The listing builds one solid part. Answer for the finished solid, in the listing's coordinates (mm). Face numbers are marked on the shaded views. Round coordinates to 2 decimals unless told otherwise and drop trailing zeros. Write each loop counter-clockwise with the first axis right and the second up, starting at its lowest first coordinate (ties: lowest second). Pieces come first, ordered by that corner, then holes.
Item 1: Find section A-A on z = 0. Give the vertices of the cut face in (x, y).
Item 2: Find section B-B on x = 0. Give the vertices of the cut face in (y, z).
Item 3: Find section C-C on y = -23. Give the vertices of the cut face in (x, z), then the cut area to 3 significant figures.
Item 4: Find section D-D on x = 38. Give the vertices of the cut face in (y, z), then the cut area to 3 significant figures.
Item 5: For a pull along Z with two mould halves and no side action, classify the marked faces 1, 2 and 3 as +Z half, -Z half, draft (parallel to the pull), parting line (faces both ways), or undercut.
Item 6: Find the intervals of material crossed by probe 1 along Z at (x, y) = (0, -11.5); probe 2 along Z at (x, y) = (-5.5, -10.5); probe 3 along X at (y, z) = (-4.5, 9), in increasing order.
Item 7: Each of these flat-tipped pins is pushed along its axis until it touches: pin 1 (4 mm diameter, centred on y = -19, z = 28, fed in from -X); pin 2 (3 mm diameter, centred on y = -14.5, z = 28, fed in from +X). Where does it stop, or does it pass through?
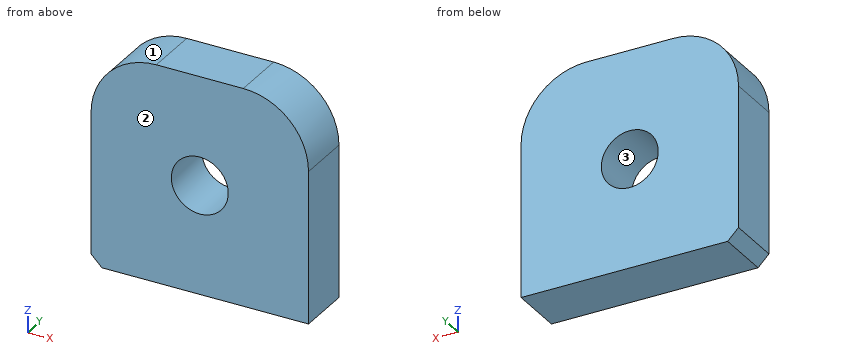
```python
from build123d import *

# Parameters (mm, degrees)
F0_W     = 100
F0_H     = 100
F1_DEPTH = 25
F2_R     = 30
F3_SIZE  = 5
F4_R     = 13.080351
F5_DEPTH = 25


with BuildPart() as f1:
    # F0 (on Front) → F1 (new body)
    with BuildSketch(Plane.XZ):
        Rectangle(F0_W, F0_H)
    extrude(amount=F1_DEPTH)

    # F2
    f2_edges = [f1.edges().sort_by_distance(p)[0] for p in [
        (-50, -12.5, 50),
        (50, -12.5, 50),
    ]]
    fillet(f2_edges, radius=F2_R)

    # F3
    f3_edges = [f1.edges().sort_by_distance(p)[0] for p in [
        (-50, -12.5, -50),
    ]]
    chamfer(f3_edges, length=F3_SIZE)

    # F4 (on face) → F5 (cut)
    with BuildSketch(Plane.XZ.offset(25)):
        Circle(F4_R)
    extrude(amount=-F5_DEPTH, mode=Mode.SUBTRACT)


solid = f1.part
```
Check values:
1. outline: (-50, -25) - (-13.08, -25) - (-13.08, 0) - (-50, 0) - close; (13.08, -25) - (50, -25) - (50, 0) - (13.08, 0) - close
2. outline: (-25, -50) - (0, -50) - (0, -13.08) - (-25, -13.08) - close; (-25, 13.08) - (0, 13.08) - (0, 50) - (-25, 50) - close
3. outline: (-50, -45) - (-45, -50) - (50, -50) - (50, 20) arc R30 ccw to (20, 50) - (-20, 50) arc R30 ccw to (-50, 20) - close; hole circle Ø26.16 at (0, 0)
3. area: 9,060 mm2
4. outline: (-25, -50) - (0, -50) - (0, 44) - (-25, 44) - close
4. area: 2,350 mm2
5. face 1: +Z half
5. face 2: draft
5. face 3: undercut
6. probe 1: z = -50 to -13.08, 13.08 to 50
6. probe 2: z = -50 to -11.87, 11.87 to 50
6. probe 3: x = -50 to -9.49, 9.49 to 50
7. pin 1: stops at x = -49.39
7. pin 2: stops at x = 49.29
